Part model, mm, in its own coordinate system. A direction names the side the tool comes from. Give positions to 0.01 mm unless a question says otherwise; leave off trailing zeros. Order: outer loops, then holes, each group sorted by start corner. A loop starts at its lowest first (then second) coordinate and runs counter-clockwise, first axis right, second up.
1. Slice it at C-C on z = -3.5. List the corners of the cut face in (x, y), and give its area (3 significant figures).
2. Which spindle directions (+Z, -Z, +X, -X, +Y, -Y) get a long thin tool onto all of the face, cutting with end or side? Do faces 5 (the cylindrical face through (48.35, 6.59, 2.43)), 6 (the flat face through (50, 7.5, -4)), 7 (the flat face through (5, 4, -4)), 8 (the cylindrical face through (12.35, 5.82, 1.7)). Say none if no direction does.
3. Drop flat-ended pins along their axis: pin 1 Ø1.5 at (x, z) = (50.5, -5) entering from +Y; pin 2 Ø4 at (x, y) = (41.75, 36.75) entering from +Z; pin 3 Ø1.9 at (x, y) = (41.75, 5.75) entering from -Z; pin 4 Ø1 at (x, y) = (44, 5.5) entering from -Z. Give the stop position or say it passes through.
4. Slice it at B-B on x = 10.75. List the corners of the cut face in (y, z).
5. Probe line 1 (Y direction, x = 41.75, z = 0.9); line 2 (Z direction, x = 50, y = 2.5); line 3 (X direction, y = 3, z = -7.5). List the from-to ranges inside material, lowest first.
6. Slice it at D-D on x = 26.25. List the corners of the cut face in (y, z).
7. Mould opens along X. For faces 1 (the cylindrical face through (23.86, 10.5, 2.46)), 2 (the cylindrical face through (0.85, 6.59, 2.43)), 3 (the flat face through (26, 42.5, 2)), 4 (the flat face through (52.5, 4, -1)) say: +X half, -X half, draft (parallel to the pull), parting line (faces both ways), or undercut.
8. Slice it at A-A on y = 5.75. List the corners of the cut face in (x, z), and give its area (3 significant figures).
from build123d import *

# Parameters (mm, degrees)
SKIZZE1_R                                            = 11.0125
AUFSATZ_LINEAR_AUSTRAGEN1_DEPTH                      = 5
AUFSATZ_LINEAR_AUSTRAGEN2_DEPTH                      = 7.5
FORMSENKUNG_F_R_M3_SENKSCHRAUBE_MIT_SCHL_D           = 3.2
FORMSENKUNG_F_R_M3_SENKSCHRAUBE_MIT_SCHL_CSINK_D     = 6.3
FORMSENKUNG_F_R_M3_SENKSCHRAUBE_MIT_SCHL_CSINK_ANGLE = 90
M4_GEWINDEBOHRUNG2_D                                 = 3.3
M4_GEWINDEBOHRUNG2_DEPTH                             = 13
M4_GEWINDEBOHRUNG2_TIP                               = 0.991420021


with BuildPart() as part:
    # Skizze1 → Aufsatz-Linear austragen1 (new body)
    with BuildSketch(Plane.XY):
        with BuildLine():
            Line((52.5, 7.5), (48.11327046, 38.207106781))
            ThreePointArc((48.11327046, 38.207106781), (46.439531698, 41.277269775), (43.163522992, 42.5))
            Line((43.163522992, 42.5), (9.336477008, 42.5))
            ThreePointArc((9.336477008, 42.5), (6.060468302, 41.277269775), (4.38672954, 38.207106781))
            Line((4.38672954, 38.207106781), (0, 7.5))
            Line((0, 7.5), (0, 0))
            Line((0, 0), (52.5, 0))
            Line((52.5, 0), (52.5, 7.5))
        make_face()
        with Locations((26.25, 21.25)):
            Circle(SKIZZE1_R, mode=Mode.SUBTRACT)
    extrude(amount=AUFSATZ_LINEAR_AUSTRAGEN1_DEPTH)

    # Skizze4 → Aufsatz-Linear austragen2 (add)
    with BuildSketch(Plane.XZ):
        with BuildLine():
            Line((52.5, 0), (47.5, 0))
            Line((47.5, 0), (47.5, -7.5))
            ThreePointArc((47.5, -7.5), (50, -10), (52.5, -7.5))
            Line((52.5, -7.5), (52.5, 0))
        make_face()
        with BuildLine():
            Line((0, 0), (5, 0))
            Line((5, 0), (5, -7.5))
            ThreePointArc((5, -7.5), (2.5, -10), (0, -7.5))
            Line((0, -7.5), (0, 0))
        make_face()
    extrude(amount=-AUFSATZ_LINEAR_AUSTRAGEN2_DEPTH)

    # Formsenkung für M3 Senkschraube mit Schlitz/Kreuzschlitz1 (through all)
    with Locations(Plane.XY.offset(5)):
        with Locations((10.75, 36.75), (41.75, 5.75), (10.75, 5.75), (41.75, 36.75)):
            CounterSinkHole(FORMSENKUNG_F_R_M3_SENKSCHRAUBE_MIT_SCHL_D / 2, FORMSENKUNG_F_R_M3_SENKSCHRAUBE_MIT_SCHL_CSINK_D / 2, counter_sink_angle=FORMSENKUNG_F_R_M3_SENKSCHRAUBE_MIT_SCHL_CSINK_ANGLE)

    # M4 Gewindebohrung2
    with Locations(Plane(origin=(0, 0, 0), x_dir=(-1, 0, 0), z_dir=(0, -1, 0))):
        with Locations((-2.5, 7.5), (-50, 7.5), (-50, -2.5), (-2.5, -2.5)):
            Hole(M4_GEWINDEBOHRUNG2_D / 2, depth=M4_GEWINDEBOHRUNG2_DEPTH)
            with Locations((0, 0, -(M4_GEWINDEBOHRUNG2_DEPTH + M4_GEWINDEBOHRUNG2_TIP / 2))):  # 118° drill point
                Cone(0, M4_GEWINDEBOHRUNG2_D / 2, M4_GEWINDEBOHRUNG2_TIP, mode=Mode.SUBTRACT)


solid = part.part
Data:
1. outline: (0, 0) - (5, 0) - (5, 7.5) - (0, 7.5) - close; (47.5, 0) - (52.5, 0) - (52.5, 7.5) - (47.5, 7.5) - close
1. area: 75.0 mm2
2. face 5: -Y
2. face 6: -Z, +X, -X, +Y
2. face 7: -Z, +Y, -Y
2. face 8: +Z, -Z
3. pin 1: stops at y = 7.5
3. pin 2: stops at z = 3.85
3. pin 3: passes through
3. pin 4: stops at z = 0
4. outline: (0, 0) - (4.15, 0) - (4.15, 3.45) - (2.6, 5) - (0, 5) - close; (7.35, 0) - (35.15, 0) - (35.15, 3.45) - (33.6, 5) - (8.9, 5) - (7.35, 3.45) - close; (38.35, 0) - (42.5, 0) - (42.5, 5) - (39.9, 5) - (38.35, 3.45) - close
5. line 1: y = 0 to 4.15, 7.35 to 35.15, 38.35 to 42.5
5. line 2: z = -10 to -9.15, -5.85 to 0.85, 4.15 to 5
5. line 3: x = 0 to 0.85, 4.15 to 5, 47.5 to 48.35, 51.65 to 52.5
6. outline: (0, 0) - (10.24, 0) - (10.24, 5) - (0, 5) - close; (32.26, 0) - (42.5, 0) - (42.5, 5) - (32.26, 5) - close
7. face 1: undercut
7. face 2: undercut
7. face 3: draft
7. face 4: +X half
8. outline: (0, -7.5) arc R2.5 ccw to (5, -7.5) - (5, 0) - (9.15, 0) - (9.15, 3.45) - (7.6, 5) - (0, 5) - close; (12.35, 0) - (40.15, 0) - (40.15, 3.45) - (38.6, 5) - (13.9, 5) - (12.35, 3.45) - close; (43.35, 0) - (47.5, 0) - (47.5, -7.5) arc R2.5 ccw to (52.5, -7.5) - (52.5, 5) - (44.9, 5) - (43.35, 3.45) - close; hole circle Ø3.3 at (2.5, -7.5); hole circle Ø3.3 at (2.5, 2.5); hole circle Ø3.3 at (50, -7.5); hole circle Ø3.3 at (50, 2.5)
8. area: 286 mm2
